```python
from build123d import *

# Parameters (mm, degrees)
SKETCH_1_W          = 29
SKETCH_1_H          = 52.5
SKETCH_1_R          = 9
EXTRUDE_1_DEPTH     = 6
SKETCH_2_W          = 6.5
SKETCH_2_H          = 3.5
CUT_EXTRUDE_1_DEPTH = 10
SKETCH_3_R          = 1
CUT_EXTRUDE_4_DEPTH = 8
SKETCH_4_R          = 1
CUT_EXTRUDE_5_DEPTH = 10


with BuildPart() as part:
    # 草图1 → 凸台-拉伸1 (new body)
    with BuildSketch(Plane(origin=(0, 0, 0), x_dir=(1, 0, 0), z_dir=(0, 1, 0))):
        Rectangle(SKETCH_1_W, SKETCH_1_H)
        with Locations(Location((0, -16.25, 0), (0, 0, 270))):
            Circle(SKETCH_1_R, mode=Mode.SUBTRACT)
        with Locations(Location((0, 9.75, 0), (0, 0, 270))):
            Circle(SKETCH_1_R, mode=Mode.SUBTRACT)
    extrude(amount=EXTRUDE_1_DEPTH)

    # 草图2 → 切除-拉伸1 (cut)
    with BuildSketch(Plane(origin=(0, 6, 0), x_dir=(1, 0, 0), z_dir=(0, 1, 0))):
        with Locations((-11.25, -24.5)):
            Rectangle(SKETCH_2_W, SKETCH_2_H)
        with Locations((11.25, -24.5)):
            Rectangle(SKETCH_2_W, SKETCH_2_H)
    extrude(amount=-CUT_EXTRUDE_1_DEPTH, mode=Mode.SUBTRACT)

    # 草图3 → 切除-拉伸4 (cut)
    with BuildSketch(Plane.XY.offset(22.75)):
        with Locations((-12, 2)):
            Circle(SKETCH_3_R)
        with Locations((12, 2)):
            Circle(SKETCH_3_R)
    extrude(amount=-CUT_EXTRUDE_4_DEPTH, mode=Mode.SUBTRACT)

    # 草图4 → 切除-拉伸5 (cut)
    with BuildSketch(Plane(origin=(0, 6, 0), x_dir=(1, 0, 0), z_dir=(0, 1, 0))):
        with Locations(Location((-11, 24.25, 0), (0, 0, 270))):
            Circle(SKETCH_4_R)
        with Locations(Location((11, 24.25, 0), (0, 0, 270))):
            Circle(SKETCH_4_R)
    extrude(amount=-CUT_EXTRUDE_5_DEPTH, mode=Mode.SUBTRACT)


solid = part.part
```
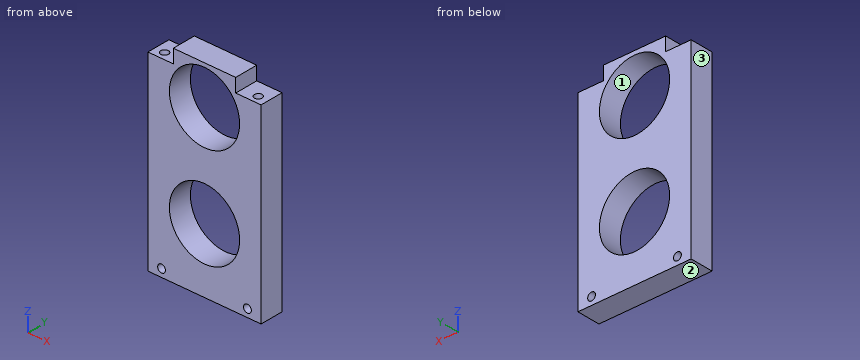
Check sheet for the modelled part. Datum: model origin and axes. Units: mm. Face numbers are marked on the shaded views. Give positions to 0.01 mm unless a question says otherwise; leave off trailing zeros. Order: outer loops, then holes, each group sorted by start corner. A loop starts at its lowest first (then second) coordinate and runs counter-clockwise, first axis right, second up. Notation, with made-up numbers: (24, 54) -> (65, 54) arc R7 ccw to (65, 66) -> close; hole circle Ø6 at (-28, 73). An arc over 180 degrees is marked (long way). Return JSON: item names as keys, results as strings.
1. Go/stop test with flat-tipped pins: P1, Ø3, axis at y = 2.5, z = 24, coming from the +X side; P2, Ø1.6, axis at x = 12.5, y = 1.5, coming from the +Z side; P3, Ø0.6, axis at x = -12, y = 1.5, coming from the +Z side; P4, Ø1, axis at y = 4.5, z = 25.5, coming from the -X side. Record where each tip stops, or that it passes through.
From the geometry:
{"P1": "x = 14.5", "P2": "z = 22.75", "P3": "z = 14.75", "P4": "x = -8"}
2. Cross-section at A-A, the plane z = 16.25. Record the cut outline in (x, y), plus the area to 3 significant figures.
From the geometry:
{"outline": "(-14.5, 0) -> (-9, 0) -> (-9, 6) -> (-14.5, 6) -> close; (9, 0) -> (14.5, 0) -> (14.5, 6) -> (9, 6) -> close; hole circle Ø2 at (-12, 2); hole circle Ø2 at (12, 2)", "area": "59.7 mm^2"}
3. Cross-section at D-D, the plane z = -9.75. Record the cut outline in (x, y).
From the geometry:
{"outline": "(-14.5, 0) -> (-9, 0) -> (-9, 6) -> (-14.5, 6) -> close; (9, 0) -> (14.5, 0) -> (14.5, 6) -> (9, 6) -> close"}
4. Cross-section at C-C, the plane x = 0. Record the cut outline in (y, z).
From the geometry:
{"outline": "(0, -26.25) -> (6, -26.25) -> (6, -18.75) -> (0, -18.75) -> close; (0, -0.75) -> (6, -0.75) -> (6, 7.25) -> (0, 7.25) -> close; (0, 25.25) -> (6, 25.25) -> (6, 26.25) -> (0, 26.25) -> close"}
5. Cross-section at B-B, the plane y = 2. Record the cut outline in (x, z).
From the geometry:
{"outline": "(-14.5, -26.25) -> (14.5, -26.25) -> (14.5, 22.75) -> (13, 22.75) -> (13, 14.75) -> (11, 14.75) -> (11, 22.75) -> (8, 22.75) -> (8, 26.25) -> (-8, 26.25) -> (-8, 22.75) -> (-11, 22.75) -> (-11, 14.75) -> (-13, 14.75) -> (-13, 22.75) -> (-14.5, 22.75) -> close; hole circle Ø2 at (-11, -24.25); hole circle Ø18 at (0, -9.75); hole circle Ø18 at (0, 16.25); hole circle Ø2 at (11, -24.25)"}
6. Mould release check, pull along X, two halves, no side actions. Record for the marked faces 1, 2 and 3: +X half, -X half, draft (parallel to the pull), parting line (faces both ways), or undercut.
From the geometry:
{"face 1": "undercut", "face 2": "draft", "face 3": "-X half"}
7. Material ranges on probe 1 along X at (y, z) = (4.8, 16.25); probe 2 along Z at (x, y) = (-5, 3.95); probe 3 along Y at (x, z) = (-12, 16.5), recorded low to high. Write a range as [from, to].
From the geometry:
{"probe 1": "[-14.5, -9], [9, 14.5]", "probe 2": "[-26.25, -17.23], [-2.27, 8.77], [23.73, 26.25]", "probe 3": "[0, 1], [3, 6]"}
